```python
from build123d import *

# Parameters (mm, degrees)
SKETCH1_R           = 5
SKETCH1_R_2         = 2.7051
BOSS_EXTRUDE1_DEPTH = 11
SKETCH2_R           = 7.5
SKETCH2_R_2         = 1.75
SKETCH2_R_3         = 1
BOSS_EXTRUDE2_DEPTH = 14
CUT_EXTRUDE1_START  = -14
SKETCH3_R           = 2.1
CUT_EXTRUDE1_DEPTH  = 6


with BuildPart() as part:
    # Sketch1 → Boss-Extrude1 (new body)
    with BuildSketch(Plane(origin=(0, 0, 0), x_dir=(1, 0, 0), z_dir=(0, 1, 0))):
        with Locations(Location((0, 0, 0), (0, 0, 270))):
            Circle(SKETCH1_R)
        with Locations(Location((0, 0, 0), (0, 0, 270))):
            Circle(SKETCH1_R_2, mode=Mode.SUBTRACT)
    extrude(amount=BOSS_EXTRUDE1_DEPTH)

    # Sketch2 → Boss-Extrude2 (add)
    with BuildSketch(Plane(origin=(0, 0, 0), x_dir=(1, 0, 0), z_dir=(0, 1, 0))):
        with Locations(Location((0, 0, 0), (0, 0, 270))):
            Circle(SKETCH2_R)
        with Locations(Location((0, 0, 0), (0, 0, 270))):
            Circle(SKETCH2_R_2, mode=Mode.SUBTRACT)
        with Locations(Location((0, 6.25, 0), (0, 0, 270))):
            Circle(SKETCH2_R_3, mode=Mode.SUBTRACT)
        with Locations(Location((6.25, 0, 0), (0, 0, 270))):
            Circle(SKETCH2_R_3, mode=Mode.SUBTRACT)
        with Locations(Location((0, -6.25, 0), (0, 0, 270))):
            Circle(SKETCH2_R_3, mode=Mode.SUBTRACT)
        with Locations(Location((-6.25, 0, 0), (0, 0, 270))):
            Circle(SKETCH2_R_3, mode=Mode.SUBTRACT)
    extrude(amount=-BOSS_EXTRUDE2_DEPTH)

    # Sketch3 → Cut-Extrude1 (cut)
    with BuildSketch(Plane(origin=(0, 0, 0), x_dir=(1, 0, 0), z_dir=(0, 1, 0)).offset(CUT_EXTRUDE1_START)):
        with Locations(Location((0, 0, 0), (0, 0, 270))):
            Circle(SKETCH3_R)
    extrude(amount=CUT_EXTRUDE1_DEPTH, mode=Mode.SUBTRACT)


solid = part.part
```
The model under review builds one solid part; all positions refer to its coordinate system, in mm. A direction names the side the tool comes from. Round coordinates to 2 decimals unless told otherwise and drop trailing zeros. Write each loop counter-clockwise with the first axis right and the second up, starting at its lowest first coordinate (ties: lowest second). Pieces come first, ordered by that corner, then holes. Notation, with made-up numbers: (76, -40) -> (120, -40) arc R14 ccw to (120, -19) -> close; hole circle Ø1 at (26, 3). An arc over 180 degrees is marked (long way). Use CSV: the item, a comma, the result in double quotes.
Q1. Consider section D-D (x = 6.25). Give the boundary of the cut face in (y, z), then the cut area to 3 significant figures.
Checks:
outline,"(-14, -4.15) -> (0, -4.15) -> (0, -1) -> (-14, -1) -> close; (-14, 1) -> (0, 1) -> (0, 4.15) -> (-14, 4.15) -> close"
area,"88.1 mm²"
Q2. To check wall thickness, follow probe 1 along X at (y, z) = (7.25, 0); probe 2 along Z at (x, y) = (0.75, -11.75); probe 3 along Y at (x, z) = (3, 5.25). State the ranges of each line that lie inside material, in increasing order. Write a range as [from, to].
Checks:
probe 1,"[-5, -2.71], [2.71, 5]"
probe 2,"[-7.46, -6.91], [-5.59, -1.96], [1.96, 5.59], [6.91, 7.46]"
probe 3,"[-14, 0]"
Q3. Consider section C-C (z = -6.25). Give the boundary of the cut face in (x, y), then the cut area to 3 significant figures.
Checks:
outline,"(-4.15, -14) -> (-1, -14) -> (-1, 0) -> (-4.15, 0) -> close; (1, -14) -> (4.15, -14) -> (4.15, 0) -> (1, 0) -> close"
area,"88.1 mm²"
Q4. Consider section B-B (x = 0). Give the boundary of the cut face in (y, z).
Checks:
outline,"(-14, -7.5) -> (0, -7.5) -> (0, -7.25) -> (-14, -7.25) -> close; (-14, -5.25) -> (0, -5.25) -> (0, -5) -> (11, -5) -> (11, -2.71) -> (0, -2.71) -> (0, -1.75) -> (-8, -1.75) -> (-8, -2.1) -> (-14, -2.1) -> close; (-14, 2.1) -> (-8, 2.1) -> (-8, 1.75) -> (0, 1.75) -> (0, 2.71) -> (11, 2.71) -> (11, 5) -> (0, 5) -> (0, 5.25) -> (-14, 5.25) -> close; (-14, 7.25) -> (0, 7.25) -> (0, 7.5) -> (-14, 7.5) -> close"
Q5. For faces 1 (the cylindrical face through (-0.61, -6.9, -7.04)), 2 (the cylindrical face through (-4.88, 5.42, -1.08)), list the 3-axis set-ups (+Z, -Z, +X, -X, +Y, -Y) from which the entire face can be reached by the end or side of a thin tool; tool diameter is ignored.
Checks:
face 1,"+Y, -Y"
face 2,"+Y"
Q6. Consider section A-A (z = 0). Give the boundary of the cut face in (x, y).
Checks:
outline,"(-7.5, -14) -> (-7.25, -14) -> (-7.25, 0) -> (-7.5, 0) -> close; (-5.25, -14) -> (-2.1, -14) -> (-2.1, -8) -> (-1.75, -8) -> (-1.75, 0) -> (-2.71, 0) -> (-2.71, 11) -> (-5, 11) -> (-5, 0) -> (-5.25, 0) -> close; (1.75, -8) -> (2.1, -8) -> (2.1, -14) -> (5.25, -14) -> (5.25, 0) -> (5, 0) -> (5, 11) -> (2.71, 11) -> (2.71, 0) -> (1.75, 0) -> close; (7.25, -14) -> (7.5, -14) -> (7.5, 0) -> (7.25, 0) -> close"
Q7. Mouldability with a two-part tool opening along X and no side actions: class faces 3 (the flat face through (-2, 0, 0)), 4 (the cylindrical face through (0.631, -11.042, 2.003)), 5 (the cylindrical face through (0.33, -6.902, -7.493)), 6 (the flat face through (-2.2, 11, 2.2)) as released by +X, released by -X, zero draft, split by the parting line, or undercut.
Checks:
face 3,"undercut"
face 4,"undercut"
face 5,"split by the parting line"
face 6,"zero draft"
Q8. For pin 1 Ø8 at (y, z) = (5.5, -5.5) entering from -X; pin 2 Ø2.5 at (x, z) = (0, -6.25) entering from -Y; pin 3 Ø3 at (x, z) = (0, 0) entering from +Y; pin 4 Ø3 at (y, z) = (-7, 2.5) entering from -X, all flat-tipped, find the tip position at first contact; note any pin that passes through.
Checks:
pin 1,"x = -4.77"
pin 2,"y = -14"
pin 3,"through"
pin 4,"x = -7.43"
